Read the model definition and answer for the solid it produces. Units are mm, in the model's axes. A direction names the side the tool comes from. Coordinates: 2 decimals unless noted, no trailing zeros. Loops run counter-clockwise (first coordinate to the right, second up) from the corner with the lowest first, then second, coordinate; pieces in that order, holes last. Notation, with made-up numbers: (-16, 46) - (1, 46) arc R22 ccw to (1, 85) - close; hole circle Ø1 at (41, 85). An arc over 180 degrees is marked (long way). Use CSV: the item, a comma, the result in double quotes.
```python
from build123d import *

# Parameters (mm, degrees)
BOSS_EXTRUDE1_DEPTH = 4.5
BOSS_EXTRUDE2_DEPTH = 3.8
BOSS_EXTRUDE3_DEPTH = 8.1
CUT_EXTRUDE2_START  = -8.1
CUT_EXTRUDE2_DEPTH  = 8.1


with BuildPart() as part:
    # Sketch1 → Boss-Extrude1 (new body)
    with BuildSketch(Plane(origin=(0, 0, 0), x_dir=(1, 0, 0), z_dir=(0, 1, 0))):
        with BuildLine():
            Line((7.25, 0), (7.25, -35))
            ThreePointArc((7.25, -35), (0, -42.25), (-7.25, -35))
            Line((-7.25, -35), (-7.25, 0))
            ThreePointArc((-7.25, 0), (0, 7.25), (7.25, 0))
        make_face()
    extrude(amount=BOSS_EXTRUDE1_DEPTH)

    # Sketch3 → Boss-Extrude2 (add)
    with BuildSketch(Plane(origin=(0, 4.5, 0), x_dir=(1, 0, 0), z_dir=(0, 1, 0))):
        with BuildLine():
            Line((-2.622571491, -0.457666807), (-2.622571491, -0.011296081))
            Line((-2.622571491, -0.011296081), (2.763792269, -0.011296081))
            Line((2.763792269, -0.011296081), (2.763792269, -0.457666807))
            ThreePointArc((2.763792269, -0.457666807), (2.791332039, -0.235236185), (2.800532634, -0.011296081))
            ThreePointArc((2.800532634, -0.011296081), (-0.153329714, 2.709425568), (-2.622571491, -0.457666807))
        make_face()
        with BuildLine():
            Line((2.763792269, -0.011296081), (-2.622571491, -0.011296081))
            Line((-2.622571491, -0.011296081), (-2.622571491, -0.457666807))
            ThreePointArc((-2.622571491, -0.457666807), (0.070610389, -2.741218326), (2.763792269, -0.457666807))
            Line((2.763792269, -0.457666807), (2.763792269, -0.011296081))
        make_face()
        with BuildLine():
            ThreePointArc((2.763792269, -0.457666807), (0.070610389, -2.741218326), (-2.622571491, -0.457666807))
            Line((-2.622571491, -0.457666807), (-2.622571491, -35.011296081))
            ThreePointArc((-2.622571491, -35.011296081), (0.070610389, -32.318114201), (2.763792269, -35.011296081))
            Line((2.763792269, -35.011296081), (2.763792269, -0.457666807))
        make_face()
        with BuildLine():
            ThreePointArc((2.763792269, -35.011296081), (0.070610389, -32.318114201), (-2.622571491, -35.011296081))
            Line((-2.622571491, -35.011296081), (2.763792269, -35.011296081))
        make_face()
        with BuildLine():
            Line((2.763792269, -35.011296081), (-2.622571491, -35.011296081))
            ThreePointArc((-2.622571491, -35.011296081), (0.070610389, -37.704477961), (2.763792269, -35.011296081))
        make_face()
    extrude(amount=BOSS_EXTRUDE2_DEPTH)

    # Sketch4 → Boss-Extrude3 (add)
    with BuildSketch(Plane(origin=(0, 8.3, 0), x_dir=(1, 0, 0), z_dir=(0, 1, 0))):
        with BuildLine():
            Line((7.25308141, 0.014627933), (7.323691799, -34.996668148))
            ThreePointArc((7.323691799, -34.996668148), (0.085238322, -42.264377491), (-7.182471021, -35.025924014))
            Line((-7.182471021, -35.025924014), (-7.25308141, -0.014627933))
            ThreePointArc((-7.25308141, -0.014627933), (-0.014627933, 7.25308141), (7.25308141, 0.014627933))
        make_face()
    extrude(amount=BOSS_EXTRUDE3_DEPTH)

    # Sketch6 → Cut-Extrude2 (cut)
    with BuildSketch(Plane(origin=(0, 16.4, 0), x_dir=(1, 0, 0), z_dir=(0, 1, 0)).offset(CUT_EXTRUDE2_START)):
        with BuildLine():
            Line((-24.579752733, 25.941605668), (4.44385737, 25.941605668))
            Line((4.44385737, 25.941605668), (4.44385737, 5.732323751))
            ThreePointArc((4.44385737, 5.732323751), (6.509808413, 3.198405594), (7.25308141, 0.014627933))
            Line((7.25308141, 0.014627933), (7.323691799, -34.996668148))
            ThreePointArc((7.323691799, -34.996668148), (6.567208075, -38.236450718), (4.44385737, -40.797669277))
            Line((4.44385737, -40.797669277), (4.44385737, -52.11567356))
            Line((4.44385737, -52.11567356), (-24.579752733, -52.11567356))
            Line((-24.579752733, -52.11567356), (-24.579752733, -65.847384837))
            Line((-24.579752733, -65.847384837), (23.383123672, -65.847384837))
            Line((23.383123672, -65.847384837), (23.383123672, 36.458721402))
            Line((23.383123672, 36.458721402), (-24.579752733, 36.458721402))
            Line((-24.579752733, 36.458721402), (-24.579752733, 25.941605668))
        make_face()
        with BuildLine():
            Line((4.44385737, 5.732323751), (4.44385737, 25.941605668))
            Line((4.44385737, 25.941605668), (-24.579752733, 25.941605668))
            Line((-24.579752733, 25.941605668), (-24.579752733, -52.11567356))
            Line((-24.579752733, -52.11567356), (4.44385737, -52.11567356))
            Line((4.44385737, -52.11567356), (4.44385737, -40.797669277))
            ThreePointArc((4.44385737, -40.797669277), (-3.154544247, -41.507893767), (-7.182471021, -35.025924014))
            Line((-7.182471021, -35.025924014), (-7.25308141, -0.014627933))
            ThreePointArc((-7.25308141, -0.014627933), (-3.198405594, 6.509808413), (4.44385737, 5.732323751))
        make_face()
        with BuildLine():
            Line((4.44385737, -40.797669277), (4.44385737, 5.732323751))
            ThreePointArc((4.44385737, 5.732323751), (-3.198405594, 6.509808413), (-7.25308141, -0.014627933))
            Line((-7.25308141, -0.014627933), (-7.182471021, -35.025924014))
            ThreePointArc((-7.182471021, -35.025924014), (-3.154544247, -41.507893767), (4.44385737, -40.797669277))
        make_face()
        with BuildLine():
            ThreePointArc((7.25308141, 0.014627933), (6.509808413, 3.198405594), (4.44385737, 5.732323751))
            Line((4.44385737, 5.732323751), (4.44385737, -40.797669277))
            ThreePointArc((4.44385737, -40.797669277), (6.567208075, -38.236450718), (7.323691799, -34.996668148))
            Line((7.323691799, -34.996668148), (7.25308141, 0.014627933))
        make_face()
    extrude(amount=CUT_EXTRUDE2_DEPTH, mode=Mode.SUBTRACT)


solid = part.part
```
Q1. Find the intervals of material crossed by probe 1 along Y at (x, z) = (-3, -1); probe 2 along X at (y, z) = (7.25, 8.5); probe 3 along Z at (x, y) = (0, 7.5), in increasing order. Write a range as [from, to].
Reported:
probe 1,"y = [0, 4.5]"
probe 2,"x = [-2.62, 2.76]"
probe 3,"z = [-2.72, 37.7]"
Q2. The part is cut by section C-C on y = 6. Determine the outline of the cut face in (x, z).
Reported:
outline,"(-2.62, 0.46) arc R2.73 ccw (long way) to (2.76, 0.46) - (2.76, 35.01) arc R2.69 ccw to (-2.62, 35.01) - close"
Q3. The part is cut by section A-A on z = 3. Determine the outline of the cut face in (x, y).
Reported:
outline,"(-7.25, 0) - (7.25, 0) - (7.25, 4.5) - (2.76, 4.5) - (2.76, 8.3) - (-2.62, 8.3) - (-2.62, 4.5) - (-7.25, 4.5) - close"
Q4. The part is cut by section D-D on y = 2. Determine the outline of the cut face in (x, z).
Reported:
outline,"(-7.25, 0) arc R7.25 ccw to (7.25, 0) - (7.25, 35) arc R7.25 ccw to (-7.25, 35) - close"
Q5. A tool of negligible diameter and unlimited length cuts with its end or side. For faces 1 (the face through (2.764, 6, 18)), 2 (the face through (7.25, 2, 17)), 3 (the face through (0.011, 6.373, 37.704)), 4 (the face through (-2.623, 6, 17)), from which of +Z, -Z, +X, -X, +Y, -Y can it reach the whole face along a straight path? Write none if from no direction.
Reported:
face 1,"+Z, +X, +Y"
face 2,"+Z, -Z, +X, +Y, -Y"
face 3,"+Z, +Y"
face 4,"+Z, -X, +Y"
Q6. Given P1, Ø3, axis at y = 7, z = 19, coming from the -X side; P2, Ø1.1, axis at y = 6.5, z = 17.5, coming from the +X side; P3, Ø3, axis at x = 5.5, z = 2, coming from the +Y side, each flat-ended and moving along its own axis, determine where each tip first touches the part or whether it passes through.
Reported:
P1,"stops at x = -2.62"
P2,"stops at x = 2.76"
P3,"stops at y = 4.5"
Q7. The part is cut by section B-B on x = -0.75. Determine the outline of the cut face in (y, z), and give its area (3 significant figures).
Reported:
outline,"(0, -7.21) - (4.5, -7.21) - (4.5, -2.59) - (8.3, -2.59) - (8.3, 37.58) - (4.5, 37.58) - (4.5, 42.21) - (0, 42.21) - close"
area,"375 mm²"
